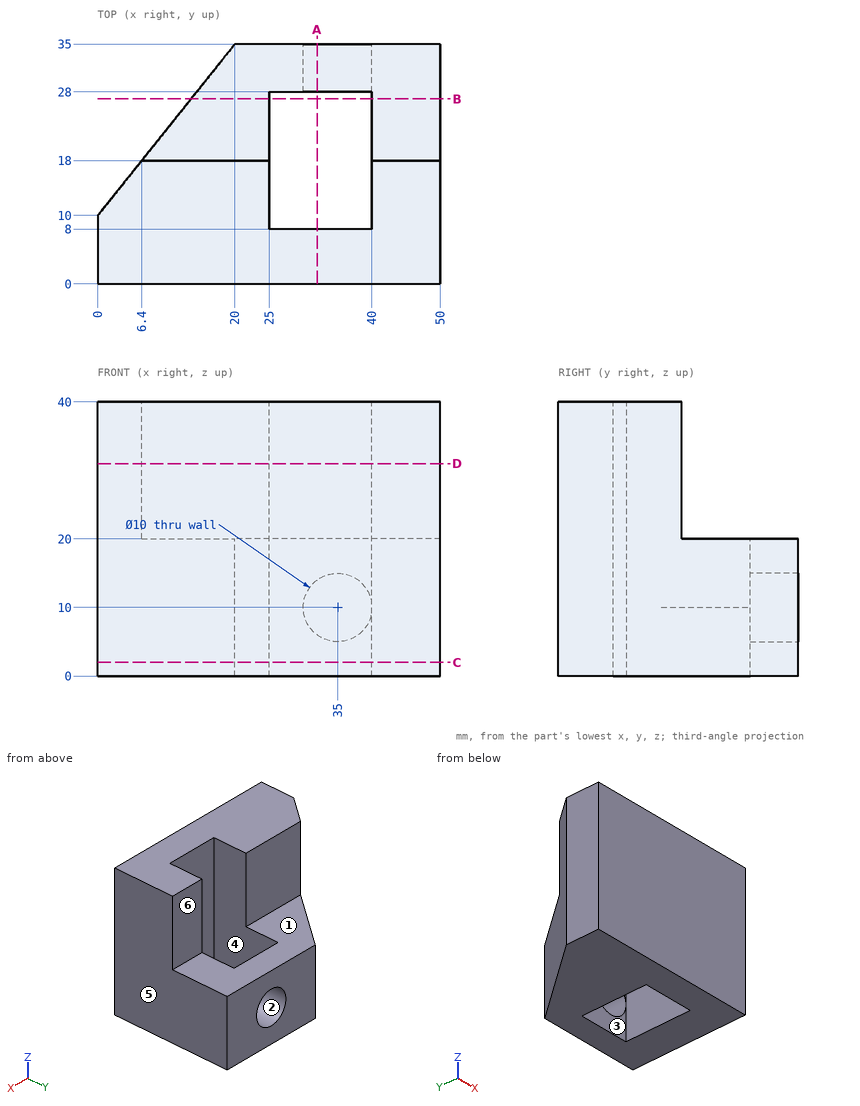
Print and shaded views of the part. All mm, measured from the part's lowest x, y and z. A direction names the side the tool comes from. Give positions to 0.01 mm unless a question says otherwise; leave off trailing zeros. Order: outer loops, then holes, each group sorted by start corner. A loop starts at its lowest first (then second) coordinate and runs counter-clockwise, first axis right, second up. Notation, with made-up numbers: (-23.75, 38.5) - (-14.75, 38.5) arc R13 ccw to (-14.75, 45.5) - close; hole circle Ø3 at (80.5, -12.5). An arc over 180 degrees is marked (long way). Use a Markdown table: item, result.
1) Saw through at C-C on z = 2. List the corners of the cut face in (x, y), plus the area to 3 significant figures.
Checked values:
| item | result |
|---|---|
| outline | (0, 0) - (50, 0) - (50, 35) - (20, 35) - (0, 10) - close; hole (25, 8) - (40, 8) - (40, 28) - (25, 28) - close |
| area | 1,200 mm² |
2) Saw through at D-D on z = 31. List the corners of the cut face in (x, y), plus the area to 3 significant figures.
Checked values:
| item | result |
|---|---|
| outline | (0, 0) - (50, 0) - (50, 18) - (40, 18) - (40, 8) - (25, 8) - (25, 18) - (6.4, 18) - (0, 10) - close |
| area | 724 mm² |
3) Saw through at B-B on y = 27. List the corners of the cut face in (x, z), plus the area to 3 significant figures.
Checked values:
| item | result |
|---|---|
| outline | (13.6, 0) - (25, 0) - (25, 20) - (13.6, 20) - close; (40, 0) - (50, 0) - (50, 20) - (40, 20) - close |
| area | 428 mm² |
4) Flat gauge pins, fed straight in: P1, Ø13.5, axis at x = 25, y = 30, coming from the +Z side; P2, Ø2, axis at x = 10, z = 8, coming from the +Y side; P3, Ø8, axis at y = 18.5, z = 13.5, coming from the -X side. Where does each tip first touch, or does it go through?
Checked values:
| item | result |
|---|---|
| P1 | z = 20 |
| P2 | y = 23.75 |
| P3 | x = 3.6 |
5) 3-axis set-ups, long thin cutter, end or side, ignore diameter. For the marked faces 1, 2 and 3: which of +Z, -Z, +X, -X, +Y, -Y reach the whole face in a straight line?
Checked values:
| item | result |
|---|---|
| face 1 | +Z, +X, -X, +Y |
| face 2 | +Y |
| face 3 | +Z, -Z |
6) Two-plate mould, pull along X, no slides. Class the marked faces 4, 5 and 6: +X half, -X half, draft (parallel to the pull), parting line (faces both ways), or undercut.
Checked values:
| item | result |
|---|---|
| face 4 | undercut |
| face 5 | +X half |
| face 6 | draft |
7) Probe L1, parallel to Y at x = 28.5, z = 8.5; L2, parallel to Z at x = 35, y = 31.75; L3, parallel to Z at x = 47, y = 25. List the from-to ranges inside material, lowest first. Write a range as from..to.
Checked values:
| item | result |
|---|---|
| L1 | 0..8, 28..35 |
| L2 | 0..5, 15..20 |
| L3 | 0..20 |
8) Saw through at A-A on x = 32. List the corners of the cut face in (y, z), plus the area to 3 significant figures.
Checked values:
| item | result |
|---|---|
| outline | (0, 0) - (8, 0) - (8, 40) - (0, 40) - close; (28, 0) - (35, 0) - (35, 6) - (28, 6) - close; (28, 14) - (35, 14) - (35, 20) - (28, 20) - close |
| area | 404 mm² |
